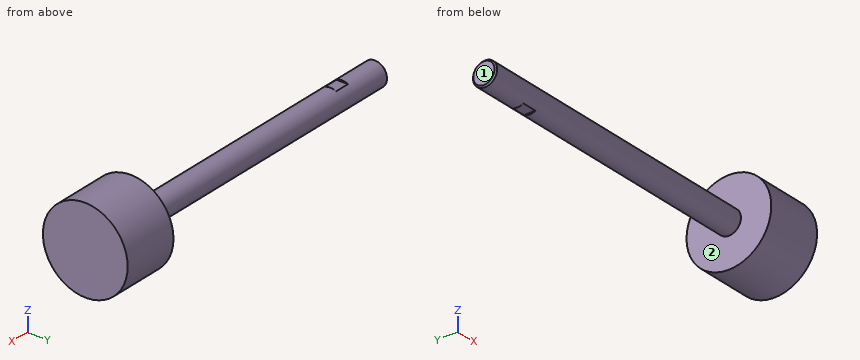
```python
from build123d import *

# Parameters (mm, degrees)
SKETCH3_W          = 25.4
SKETCH3_H          = 25.4
SKETCH3_W_2        = 11.176
SKETCH3_H_2        = 12.7
CUT_EXTRUDE1_DEPTH = 7.874


with BuildPart() as part:
    # Sketch1 → Revolve1 (revolve)
    with BuildSketch(Plane.XY):
        Polygon((-7.874, 0), (-7.874, 6.35), (131.445, 6.35), (131.445, 22.34565), (161.671, 22.34565), (161.671, 0), align=None)
    revolve(axis=Axis((161.671, 0, 0), (-1, 0, 0)))

    # Sketch2 → Revolve2 (revolve)
    with BuildSketch(Plane.XY):
        Polygon((-30.226, 0), (-30.226, 5.59435), (-29.47035, 6.35), (-7.874, 6.35), (-7.874, 0), align=None)
    revolve(axis=Axis((-7.874, 0, 0), (-1, 0, 0)))

    # Sketch3 → Cut-Extrude1 (cut)
    with BuildSketch(Plane(origin=(-7.874, 0, 0), x_dir=(0, 0, -1), z_dir=(1, 0, 0))):
        Rectangle(SKETCH3_W, SKETCH3_H)
        Rectangle(SKETCH3_W_2, SKETCH3_H_2, mode=Mode.SUBTRACT)
    extrude(amount=CUT_EXTRUDE1_DEPTH, mode=Mode.SUBTRACT)


solid = part.part
```
Can you work these out from the model? Positions are in its coordinate system, mm. Face numbers are marked on the shaded views. A direction names the side the tool comes from. Coordinates: 2 decimals unless noted, no trailing zeros. Order: outer loops, then holes, each group sorted by start corner. A loop starts at its lowest first (then second) coordinate and runs counter-clockwise, first axis right, second up. Notation, with made-up numbers: (55.5, 22.25) - (112.5, 22.25) arc R19 ccw to (112.5, 53.25) - close; hole circle Ø11 at (81.5, 27). An arc over 180 degrees is marked (long way). Answer in a Markdown table with one row per item.
1. Suppose I cut it at C-C (x = 53). Please give me the cut outline in (y, z).
Reply:
| item | result |
|---|---|
| outline | circle Ø12.7 at (0, 0) |
2. Suppose I cut it at B-B (z = 0). Please give me the cut outline in (x, y) (3 decimals).
Reply:
| item | result |
|---|---|
| outline | (-30.226, -5.594) - (-29.47, -6.35) - (131.445, -6.35) - (131.445, -22.346) - (161.671, -22.346) - (161.671, 22.346) - (131.445, 22.346) - (131.445, 6.35) - (-29.47, 6.35) - (-30.226, 5.594) - close |
3. For pin 1 (1 mm diameter, centred on y = -11, z = 11, fed in from -X) (3 decimals); pin 2 (1 mm diameter, centred on x = 69.5, y = -6, fed in from +Z); pin 3 (8 mm diameter, centred on x = 67, y = 11, fed in from -Z); pin 4 (6.5 mm diameter, centred on x = -5, y = -0.5, fed in from +Z), each with a flat end and sliding along its axis, tell me the tip position at first contact or that it passes through.
Reply:
| item | result |
|---|---|
| pin 1 | stops at x = 131.445 |
| pin 2 | stops at z = 3.17 |
| pin 3 | passes through |
| pin 4 | stops at z = 6.35 |
4. Suppose I cut it at A-A (y = 0). Please give me the cut outline in (x, z) (3 decimals).
Reply:
| item | result |
|---|---|
| outline | (-30.226, -5.594) - (-29.47, -6.35) - (-7.874, -6.35) - (-7.874, -5.588) - (0, -5.588) - (0, -6.35) - (131.445, -6.35) - (131.445, -22.346) - (161.671, -22.346) - (161.671, 22.346) - (131.445, 22.346) - (131.445, 6.35) - (0, 6.35) - (0, 5.588) - (-7.874, 5.588) - (-7.874, 6.35) - (-29.47, 6.35) - (-30.226, 5.594) - close |
5. If I drill on line 1 along X through (y, z) = (3.5, 13.5) (3 decimals); line 2 along Y through (x, z) = (29, 0); line 3 along Y through (x, z) = (145.5, 6), over which ranges is the centre line in solid material (lowest first)?
Reply:
| item | result |
|---|---|
| line 1 | x = 131.445 to 161.671 |
| line 2 | y = -6.35 to 6.35 |
| line 3 | y = -21.53 to 21.53 |
6. For the marked faces 1 and 2, which set-ups out of +Z, -Z, +X, -X, +Y, -Y let a thin tool reach every point of the face, with its end or its side?
Reply:
| item | result |
|---|---|
| face 1 | +Z, -Z, -X, +Y, -Y |
| face 2 | -X |
7. Suppose I cut it at D-D (z = 13). Please give me the cut outline in (x, y) (3 decimals).
Reply:
| item | result |
|---|---|
| outline | (131.445, -18.175) - (161.671, -18.175) - (161.671, 18.175) - (131.445, 18.175) - close |
